Geometry: final body of the model. Coordinates: model frame, mm. Round coordinates to 2 decimals unless told otherwise and drop trailing zeros. Write each loop counter-clockwise with the first axis right and the second up, starting at its lowest first coordinate (ties: lowest second). Pieces come first, ordered by that corner, then holes. Notation, with made-up numbers: M 56.25,71 L 76.25,71 A13 ccw 76.25,75 Z; hole C 73,-23 d7. An arc over 180 degrees is marked long. Use one line per item in the form item = value. Start each with the question number.
Item 1: Pull-direction query (Y, two-part tool) for faces 1 (the flat face through (2, 11, 0)), 2 (the cylindrical face through (1.774, 15.235, -5.522)), 3 (the flat face through (2, 18, -11)); classes: pulls with the +Y half, pulls with the -Y half, needs draft (parallel to the pull), parting line crosses it, or undercut.
Item 2: Section query C-C (x = 1.05). Return loops of the section in (y, z).
Item 3: Section query A-A (y = 13.5). Return loops of the section in (x, z), and give its area (3 significant figures).
Item 4: Section query D-D (z = -13). Return loops of the section in (x, y), and give its area (4 significant figures).
Item 5: Section query B-B (z = -17.25). Return loops of the section in (x, y).
Item 6: Ray query, probe 1 along Z at (x, y) = (2.2, 13); probe 2 along Z at (x, y) = (0.35, 14.25); probe 3 along X at (y, z) = (4.5, -5.5). Return the intervals inside material, ascending.
from build123d import *

# Parameters (mm, degrees)
SKETCH1_W           = 23
SKETCH1_H           = 18
BOSS_EXTRUDE1_DEPTH = 3.5
CUT_EXTRUDE1_DEPTH  = 30.41513216
SKETCH3_R           = 1.75
CUT_EXTRUDE3_DEPTH  = 30.41513216


with BuildPart() as part:
    # Sketch1 → Boss-Extrude1 (new body)
    with BuildSketch(Plane(origin=(0, 0, 0), x_dir=(0, 0, -1), z_dir=(1, 0, 0))):
        with Locations((11.5, 9)):
            Rectangle(SKETCH1_W, SKETCH1_H)
    extrude(amount=BOSS_EXTRUDE1_DEPTH)

    # Sketch2 → Cut-Extrude1 (cut, through all)
    with BuildSketch(Plane.XY):
        Polygon((3.5, 9), (0, 0), (3.5, 0), align=None)
    extrude(amount=-CUT_EXTRUDE1_DEPTH, mode=Mode.SUBTRACT)

    # Sketch3 → Cut-Extrude3 (cut, through all)
    with BuildSketch(Plane(origin=(3.5, 0, 0), x_dir=(0, 0, -1), z_dir=(1, 0, 0))):
        with Locations((5.75, 13.5)):
            Circle(SKETCH3_R)
        with Locations((17.25, 13.5)):
            Circle(SKETCH3_R)
    extrude(amount=-CUT_EXTRUDE3_DEPTH, mode=Mode.SUBTRACT)


solid = part.part
Working result:
q1.face_1 = needs draft
q1.face_2 = undercut
q1.face_3 = pulls with the +Y half
q2.outline = M 2.7,-23 L 18,-23 L 18,0 L 2.7,0 Z; hole C 13.5,-17.25 d3.5; hole C 13.5,-5.75 d3.5
q3.outline = M 0,-23 L 3.5,-23 L 3.5,-19 L 0,-19 Z; M 0,-15.5 L 3.5,-15.5 L 3.5,-7.5 L 0,-7.5 Z; M 0,-4 L 3.5,-4 L 3.5,0 L 0,0 Z
q3.area = 56.0 mm²
q4.outline = M 0,0 L 3.5,9 L 3.5,18 L 0,18 Z
q4.area = 47.25 mm²
q5.outline = M 0,0 L 3.5,9 L 3.5,11.75 L 0,11.75 Z; M 0,15.25 L 3.5,15.25 L 3.5,18 L 0,18 Z
q6.probe_1 = -23 to -18.93, -15.57 to -7.43, -4.07 to 0
q6.probe_2 = -23 to -18.83, -15.67 to -7.33, -4.17 to 0
q6.probe_3 = 0 to 1.75
